Part print with two shaded views. Sizes in mm from the minimum x, y, z corner. A direction names the side the tool comes from. Round coordinates to 2 decimals unless told otherwise and drop trailing zeros. Order: outer loops, then holes, each group sorted by start corner. A loop starts at its lowest first (then second) coordinate and runs counter-clockwise, first axis right, second up. Notation, with made-up numbers: M 86,23 L 90,23 A18 cw 90,53 Z; hole C 46.25,-23 d8. An arc over 180 degrees is marked long. Put each result on its own line as item: value.
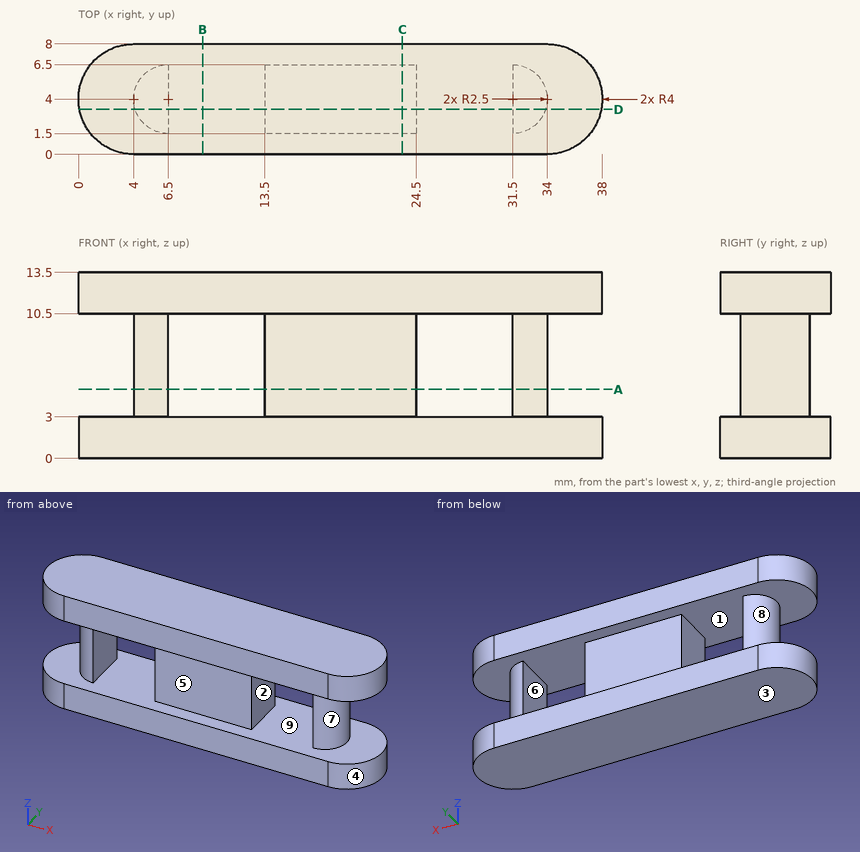
Item 1: Band-saw the part on A-A on z = 5. Give the cut face in (x, y), and give its area (3 significant figures).
Answers below:
outline: M 6.5,1.5 L 6.5,6.5 A2.5 ccw Z; M 13.5,1.5 L 24.5,1.5 L 24.5,6.5 L 13.5,6.5 Z; M 31.5,1.5 A2.5 ccw 31.5,6.5 Z
area: 74.6 mm²
Item 2: Band-saw the part on C-C on x = 23.5. Give the cut face in (y, z).
Answers below:
outline: M 0,0 L 8,0 L 8,3 L 6.5,3 L 6.5,10.5 L 8,10.5 L 8,13.5 L 0,13.5 L 0,10.5 L 1.5,10.5 L 1.5,3 L 0,3 Z
Item 3: Probe line 1 along Z through (x, y) = (4, 0.5); line 2 along X through (y, z) = (2.25, 5); line 3 along X through (y, z) = (4.25, 7.5). List the from-to ranges inside material, lowest first. Write a range as [from, to].
Answers below:
line 1: [0, 3], [10.5, 13.5]
line 2: [4.71, 6.5], [13.5, 24.5], [31.5, 33.29]
line 3: [4.01, 6.5], [13.5, 24.5], [31.5, 33.99]
Item 4: Band-saw the part on D-D on y = 3.25. Give the cut face in (x, z).
Answers below:
outline: M 0.07,0 L 37.93,0 L 37.93,3 L 33.88,3 L 33.88,10.5 L 37.93,10.5 L 37.93,13.5 L 0.07,13.5 L 0.07,10.5 L 4.12,10.5 L 4.12,3 L 0.07,3 Z; hole M 6.5,3 L 13.5,3 L 13.5,10.5 L 6.5,10.5 Z; hole M 24.5,3 L 31.5,3 L 31.5,10.5 L 24.5,10.5 Z
Item 5: Tool access for the marked faces 5, 6, 7, 8 and 9: list every direction of +Z, -Z, +X, -X, +Y, -Y with a clear straight run to the whole face (end or side of a thin tool).
Answers below:
face 5: +X, -X, -Y
face 6: +Y, -Y
face 7: +X
face 8: -X
face 9: none
Item 6: Mould opens along X. For the marked faces 1, 2, 3 and 4 say: pulls with the +X half, pulls with the -X half, needs draft (parallel to the pull), parting line crosses it, or undercut.
Answers below:
face 1: undercut
face 2: undercut
face 3: needs draft
face 4: pulls with the +X half
Item 7: Band-saw the part on B-B on x = 9. Give the cut face in (y, z).
Answers below:
outline: M 0,0 L 8,0 L 8,3 L 0,3 Z; M 0,10.5 L 8,10.5 L 8,13.5 L 0,13.5 Z
Item 8: Pin check, flat tips, straight feed: P1, Ø4, axis at y = 4.5, z = 6.5, coming from the +X side; P2, Ø1.5, axis at y = 7, z = 5, coming from the -X side; P3, Ø4, axis at y = 6, z = 6.5, coming from the -X side. Stop position of each tip, or through.
Answers below:
P1: x = 34
P2: x = 5.41
P3: x = 4
